Autodesk Inventor part; units mm, degrees
ref_plane "1_to_k_XY" through (0.5, 0, 0) normal (1, 0, 0) x (0, 0, -1)
ref_plane "1_to_k_YZ" through (0.5, 0, 0) normal (0, 0, -1) x (0, 1, 0)
ref_plane "1_to_k_ZX" through (0.5, 0, 0) normal (0, 1, 0) x (1, 0, 0)
sketch "Sketch_2" plane through (0, 0, 0) normal (0, 0, 1) x (1, 0, 0)
  line L0 (4, 0) -> (0, 0)
  line L1 (0, 0) -> (0, 5.75)
  line L2 (0, 5.75) -> (3, 7.5)
  line L3 (3, 7.5) -> (4, 7.5)
  line L4 (4, 7.5) -> (4, 0)
  line L5 (4, 0) -> (0, 0)
revolve "Revolution1" add sketch "Sketch_2" angle 360 about axis through (4, 0, 0) along (1, 0, 0)
sketch "Sketch_5" plane through (0, 0, 0) normal (0, 0, 1) x (1, 0, 0)
  line L0 (12.5, 0) -> (4, 0)
  line L1 (4, 0) -> (4, 6)
  line L2 (4, 6) -> (11.8865, 6)
  line L3 (11.8865, 6) -> (12.5, 5.3865)
  line L4 (12.5, 5.3865) -> (12.5, 0)
  line L5 (12.5, 0) -> (4, 0)
revolve "Revolution2" add sketch "Sketch_5" angle 360 about axis through (12.5, 0, 0) along (1, 0, 0)
thread "Thread1"
sketch "Sketch_13" plane through (12.5, 0, 0) normal (1, 0, 0) x (0, 0, -1)
  line L0 (-10, -20) -> (10, -20)
  line L1 (10, -20) -> (10, 20)
  line L2 (10, 20) -> (-10, 20)
  line L3 (-10, 20) -> (-10, -20)
  line L4 (-5.35, -10) -> (5.35, -10)
  line L5 (5.35, -10) -> (5.35, 10)
  line L6 (5.35, 10) -> (-5.35, 10)
  line L7 (-5.35, 10) -> (-5.35, -10)
extrude "Extrusion1" cut sketch "Sketch_13" against normal blind 8.5
sketch "Sketch_1" plane through (0, 0, 0) normal (0, 0, 1) x (1, 0, 0)
  line L0 (8, 0) -> (5, 0)
  line L1 (5, 0) -> (5, 7.5)
  line L2 (5, 7.5) -> (5.4019, 9)
  line L3 (5.4019, 9) -> (7.5981, 9)
  line L4 (7.5981, 9) -> (8, 7.5)
  line L5 (8, 7.5) -> (8, 0)
  line L6 (8, 0) -> (5, 0)
revolve "Revolution3" add sketch "Sketch_1" angle 360 about axis through (8, 0, 0) along (1, 0, 0)
sketch "Sketch_4" plane through (0, 0, 0) normal (0, 0, 1) x (1, 0, 0)
  line L0 (11, 0) -> (8, 0)
  line L1 (8, 0) -> (8, 7.5)
  line L2 (8, 7.5) -> (8.4019, 9)
  line L3 (8.4019, 9) -> (10.5981, 9)
  line L4 (10.5981, 9) -> (11, 7.5)
  line L5 (11, 7.5) -> (11, 0)
  line L6 (11, 0) -> (8, 0)
revolve "Revolution4" add sketch "Sketch_4" angle 360 about axis through (11, 0, 0) along (1, 0, 0)
sketch "Sketch_3" plane through (5, 0, 0) normal (1, 0, 0) x (0, 0, -1)
  line L0 (-15, -15) -> (15, -15)
  line L1 (15, -15) -> (15, 15)
  line L2 (15, 15) -> (-15, 15)
  line L3 (-15, 15) -> (-15, -15)
  line L4 (-7.5, 4.3301) -> (-7.5, -4.3301)
  line L5 (-7.5, -4.3301) -> (0, -8.6603)
  line L6 (0, -8.6603) -> (7.5, -4.3301)
  line L7 (7.5, -4.3301) -> (7.5, 4.3301)
  line L8 (7.5, 4.3301) -> (0, 8.6603)
  line L9 (0, 8.6603) -> (-7.5, 4.3301)
extrude "Extrusion2" cut sketch "Sketch_3" along normal blind 6
sketch "Sketch_7" plane through (0, 0, 0) normal (1, 0, 0) x (0, 1, 0)
  circle A0 centre (0, 0) radius 3.707
extrude "Extrusion3" cut sketch "Sketch_7" along normal blind 12.5
sketch "Sketch_6" plane through (0, 0, 0) normal (0, 0, 1) x (1, 0, 0)
  line L0 (14.5, 0) -> (12.5, 0)
  line L1 (12.5, 0) -> (12.5, 5.35)
  line L2 (12.5, 5.35) -> (14.5, 5.35)
  line L3 (14.5, 5.35) -> (14.5, 0)
  line L4 (14.5, 0) -> (12.5, 0)
revolve "Revolution5" add sketch "Sketch_6" angle 360 about axis through (14.5, 0, 0) along (1, 0, 0)
sketch "Sketch_8" plane through (0, 0, 0) normal (0, 0, 1) x (1, 0, 0)
  line L0 (14.5, 0) -> (12.5, 0)
  line L1 (12.5, 0) -> (12.5, 1.5)
  line L2 (12.5, 1.5) -> (12.7705, 1.2295)
  line L3 (12.7705, 1.2295) -> (14.2295, 1.2295)
  line L4 (14.2295, 1.2295) -> (14.5, 1.5)
  line L5 (14.5, 1.5) -> (14.5, 0)
  line L6 (14.5, 0) -> (12.5, 0)
revolve "Revolution6" cut sketch "Sketch_8" angle 360 about axis through (14.5, 0, 0) along (1, 0, 0)
thread "Thread2"
sketch "Sketch_9" plane through (0, 0, 0) normal (1, 0, 0) x (0, 1, 0)
  line L0 (0, 0.55) -> (0, -0.55)
  line L1 (0, -0.55) -> (4.6009, -0.55)
  line L2 (4.6009, -0.55) -> (4.6009, 0.55)
  line L3 (4.6009, 0.55) -> (0, 0.55)
extrude "Extrusion4" cut sketch "Sketch_9" along normal blind 0.5
sketch "Sketch_10" plane through (0, 0, 0) normal (1, 0, 0) x (0, 1, 0)
  line L0 (0.55, 4.6009) -> (-0.55, 4.6009)
  line L1 (-0.55, 4.6009) -> (-0.55, 0)
  line L2 (-0.55, 0) -> (0.55, 0)
  line L3 (0.55, 0) -> (0.55, 4.6009)
extrude "Extrusion5" cut sketch "Sketch_10" along normal blind 0.5
sketch "Sketch_14" plane through (14.5, 0, 0) normal (1, 0, 0) x (0, 0, -1)
  line L0 (-5, 19) -> (-5, 2.5)
  line L1 (-5, 2.5) -> (-3.1225, 2.5)
  arc A0 (-3.1225, 2.5) -> (2.5, -3.1225) centre (0, 0) ccw
  line L2 (2.5, -3.1225) -> (2.5, -4.73)
  arc A1 (2.5, -4.73) -> (5, -1.9033) centre (0, 0) ccw
  line L3 (5, -1.9033) -> (5, 19)
  arc A2 (5, 19) -> (-5, 19) centre (0, 19) ccw
extrude "Extrusion6" add sketch "Sketch_14" along normal blind 1.6
sketch "Sketch_15" plane through (0, 0, 0) normal (0, 0, 1) x (1, 0, 0)
  line L0 (18.8, 0) -> (16.1, 0)
  line L1 (16.1, 0) -> (16.1, 3)
  line L2 (16.1, 3) -> (16.4, 3)
  line L3 (16.4, 3) -> (16.4, 2.5)
  line L4 (16.4, 2.5) -> (17.607, 2.5)
  arc A0 (18.8, 0.5) -> (17.607, 2.5) centre (16.692, 0.5984) ccw
  line L5 (18.8, 0.5) -> (18.8, 0)
  line L6 (18.8, 0) -> (16.1, 0)
revolve "Revolution7" add sketch "Sketch_15" angle 360 about axis through (18.8, 0, 0) along (1, 0, 0)
ref_plane "1_to_k_XY" through (0.5, 0, 0) normal (1, 0, 0) x (0, 0, -1)
ref_plane "1_to_k_YZ" through (0.5, 0, 0) normal (0, 0, -1) x (0, 1, 0)
ref_plane "1_to_k_ZX" through (0.5, 0, 0) normal (0, 1, 0) x (1, 0, 0)
ref_plane "1_TO_2_XY" through (0, 0, 0) normal (1, 0, 0) x (0, 0, -1)
ref_plane "1_TO_2_YZ" through (0, 0, 0) normal (0, 0, -1) x (0, 1, 0)
ref_plane "1_TO_2_ZX" through (0, 0, 0) normal (0, 1, 0) x (1, 0, 0)
properties part number "LOCNL2_1"
Source: CAD feature listing. Evaluate the final solid. Frame: model axes, mm. A direction names the side the tool comes from. Give positions to 0.01 mm unless a question says otherwise; leave off trailing zeros. Loops run counter-clockwise (first coordinate to the right, second up) from the corner with the lowest first, then second, coordinate; pieces in that order, holes last. Notation, with made-up numbers: (29, -12.5) -> (80, -12.5) arc R10 ccw to (80, -6.5) -> close; hole circle Ø10 at (-26, -38.75). An arc over 180 degrees is marked (long way). Use a Markdown table: item, result. Add a question column.
(1) Section query B-B (x = 2). Output: boundary loops of the cut face in (y, z).
(2) Access query for faces 1 (the face through (6.16, -2.73, -2.51)), 2 (the face through (6.479, 6.465, -3.803)), 3 (the face through (15, 8, -5)). Directions: +Z, -Z, +X, -X, +Y, -Y. A direction counts if a zero-diameter tool reaches every point of the face in a straight line with its end or side. Return the directions, or none.
(3) Ray query, line 1 (Z direction, x = 7.25, y = 0); line 2 (Z direction, x = 13.15, y = 0); line 3 (Y direction, x = 4.75, z = 0). Return the intervals inside material, ascending.
(4) Pull-direction query (Y, two-part tool) for faces 4 (the face through (15.289, -2.886, 2.77)), 5 (the face through (9.479, 6.526, 3.698)), 6 (the face through (15.29, -3.52, -4.03)); classes: +Y half, -Y half, draft (parallel to the pull), parting line (faces both ways), or undercut.
(5) First-contact query: pin 1 Ø1 at (y, z) = (4.5, 1) entering from +X; pin 2 Ø4 at (y, z) = (14.5, -3) entering from -X; pin 3 Ø5 at (x, y) = (15.5, -1) entering from +Z. Flat tips, straight axial feed; report the tip coordinate or a pass-through.
(6) Section query A-A (y = 14). Output: boundary loops of the cut face in (x, z).
Checked values:
| question | item | result |
|---|---|---|
| 1 | outline | circle Ø13.83 at (0, 0); hole circle Ø7.41 at (0, 0) |
| 2 | face 1 | -X |
| 2 | face 2 | -Z, -X, +Y |
| 2 | face 3 | -Z, +X, +Y, -Y |
| 3 | line 1 | -7.5 to -3.71, 3.71 to 7.5 |
| 3 | line 2 | -5.35 to -1.23, 1.23 to 5.35 |
| 3 | line 3 | -6 to -3.71, 3.71 to 6 |
| 4 | face 4 | undercut |
| 4 | face 5 | +Y half |
| 4 | face 6 | -Y half |
| 5 | pin 1 | x = 16.1 |
| 5 | pin 2 | x = 14.5 |
| 5 | pin 3 | z = 5.35 |
| 6 | outline | (14.5, -5) -> (16.1, -5) -> (16.1, 5) -> (14.5, 5) -> close |
